from build123d import *

# Parameters (mm, degrees)
F1_DEPTH       = 40
F2_R           = 8
F3_R           = 5
F5_D           = 4.2
F5_CSINK_D     = 8
F5_CSINK_ANGLE = 90
F6_SIZE        = 4.99999


# Not quite as in the source:
# - a fillet or chamfer is up to 0.001 mm smaller than in the source, because OpenCascade refuses the exact size


with BuildPart() as f1:
    # F0 (on Front) → F1 (new body)
    with BuildSketch(Plane.XZ):
        Polygon((-73, 10), (-73, 0), (0, 0), (73, 0), (73, 10), (55, 10), (55, 107), (60, 107), (60, 117), (0, 117), (-60, 117), (-60, 107), (-55, 107), (-55, 10), align=None)
        Polygon((0, 10), (-40, 10), (0, 50), (40, 10), align=None, mode=Mode.SUBTRACT)
        Polygon((-9, 59), (-40, 28), (-40, 90), align=None, mode=Mode.SUBTRACT)
        Polygon((40, 90), (40, 28), (9, 59), align=None, mode=Mode.SUBTRACT)
        Polygon((40, 108), (0, 68), (-40, 108), (0, 108), align=None, mode=Mode.SUBTRACT)
    extrude(amount=F1_DEPTH)

    # F2
    f2_edges = [f1.edges().sort_by_distance(p)[0] for p in [
        (-40, -20, 108),
        (40, -20, 108),
    ]]
    fillet(f2_edges, radius=F2_R)

    # F3
    f3_edges = [f1.edges().sort_by_distance(p)[0] for p in [
        (-40, -20, 10),
        (40, -20, 10),
    ]]
    fillet(f3_edges, radius=F3_R)

    # F5 (through all)
    with Locations(Plane.XY.offset(10)):
        with Locations((-65.8, -9.9), (-65.8, -30.1), (65.8, -30.1), (65.8, -9.9)):
            CounterSinkHole(F5_D / 2, F5_CSINK_D / 2, counter_sink_angle=F5_CSINK_ANGLE)

    # F6 (size 5 in the source; OpenCascade refuses exactly that, so slightly less here)
    f6_edges = [f1.edges().sort_by_distance(p)[0] for p in [
        (-55, -20, 107),
        (55, -20, 107),
    ]]
    chamfer(f6_edges, length=F6_SIZE)


solid = f1.part
Part model, mm, in its own coordinate system. A direction names the side the tool comes from. Give positions to 0.01 mm unless a question says otherwise; leave off trailing zeros. Write each loop counter-clockwise with the first axis right and the second up, starting at its lowest first coordinate (ties: lowest second). Pieces come first, ordered by that corner, then holes.
1) Cut at A-A on x = 17.5. Write the cut outline in (y, z), then the cut area to 3 significant figures.
Resolved:
outline: (-40, 0) - (0, 0) - (0, 10) - (-40, 10) - close; (-40, 32.5) - (0, 32.5) - (0, 50.5) - (-40, 50.5) - close; (-40, 67.5) - (0, 67.5) - (0, 85.5) - (-40, 85.5) - close; (-40, 108) - (0, 108) - (0, 117) - (-40, 117) - close
area: 2,200 mm2
2) Cut at D-D on x = -34.5. Write the cut outline in (y, z), then the cut area to 3 significant figures.
Resolved:
outline: (-40, 0) - (0, 0) - (0, 33.5) - (-40, 33.5) - close; (-40, 84.5) - (0, 84.5) - (0, 117) - (-40, 117) - close
area: 2,640 mm2
3) Cut at B-B on z = 44. Write the cut outline in (x, y), then the cut area to 3 significant figures.
Resolved:
outline: (-55, -40) - (-40, -40) - (-40, 0) - (-55, 0) - close; (-24, -40) - (-6, -40) - (-6, 0) - (-24, 0) - close; (6, -40) - (24, -40) - (24, 0) - (6, 0) - close; (40, -40) - (55, -40) - (55, 0) - (40, 0) - close
area: 2,640 mm2
4) Cut at C-C on x = -65.8. Write the cut outline in (y, z), then the cut area to 3 significant figures.
Resolved:
outline: (-40, 0) - (-32.2, 0) - (-32.2, 8.1) - (-34.1, 10) - (-40, 10) - close; (-28, 0) - (-12, 0) - (-12, 8.1) - (-13.9, 10) - (-26.1, 10) - (-28, 8.1) - close; (-7.8, 0) - (0, 0) - (0, 10) - (-5.9, 10) - (-7.8, 8.1) - close
area: 309 mm2
5) Pin check, flat tips, straight feed: pin 1 (1 mm diameter, centred on y = -29, z = 51.5, fed in from +X); pin 2 (5.5 mm diameter, centred on x = -65.8, y = -9.9, fed in from -Z); pin 3 (12 mm diameter, centred on y = -19.5, z = 72, fed in from -X); pin 4 (5 mm diameter, centred on x = 65.8, y = -9.9, fed in from +Z). Stop position of each tip, or through.
Resolved:
pin 1: stops at x = 55
pin 2: stops at z = 0
pin 3: stops at x = -55
pin 4: stops at z = 8.5
6) Two-plate mould, pull along Z, no slides. Class faces 1 (the face through (-1, -20, 0)), 2 (the face through (67.9, -9.81, 3.99)), 3 (the face through (24, -20, 74)), 4 (the face through (-32.516, -20.28, 13.011)): released by +Z, released by -Z, zero draft, split by the parting line, or undercut.
Resolved:
face 1: released by -Z
face 2: zero draft
face 3: undercut
face 4: undercut
7) Probe L1, parallel to X at y = -30.1, z = 6.25; L2, parallel to Y at x = 65.8, z = 4.5; L3, parallel to Z at x = -13, y = -19.5. List the from-to ranges inside material, lowest first.
Resolved:
L1: x = -73 to -67.9, -63.7 to 63.7, 67.9 to 73
L2: y = -40 to -32.2, -28 to -12, -7.8 to 0
L3: z = 0 to 10, 37 to 55, 63 to 81, 108 to 117
8) Which spindle directions (+Z, -Z, +X, -X, +Y, -Y) get a long thin tool onto all of the face, cutting with end or side? Do faces 5 (the face through (-64, -20, 10)), 6 (the face through (-24, -20, 44)), 7 (the face through (-60, -20, 112)). Say none if no direction does.
Resolved:
face 5: -X, +Y, -Y
face 6: +Y, -Y
face 7: +Z, -X, +Y, -Y
